The model under review builds one solid part; all positions refer to its coordinate system, in mm. Give positions to 0.01 mm unless a question says otherwise; leave off trailing zeros. Loops run counter-clockwise (first coordinate to the right, second up) from the corner with the lowest first, then second, coordinate; pieces in that order, holes last. Notation, with made-up numbers: (41, 57.25) -> (64, 57.25) arc R14 ccw to (64, 74.25) -> close; hole circle Ø3 at (-19.5, -33.75). An arc over 180 degrees is marked (long way). Write each question's results on one line, items separated by ' | '. Start each with the question number.
Q1. Insertion check: pin 1 Ø2.5 at (y, z) = (4, 0.5) entering from -X; pin 2 Ø4 at (x, y) = (116, 0) entering from -Z. Each pin has a flat end and moves straight along its axis. Give the tip position at first contact, or say it passes through.
Q2. Wall thickness on L1, parallel to X at y = 0, z = 3.35; L2, parallel to X at y = 1, z = 3.85; L3, parallel to Y at x = 116, z = 3.15: over which ranges is each line inside the solid? List them lowest first. Write a range as [from, to].
Q3. We need section A-A (z = 1.35). Write out the cut boundary in (x, y).
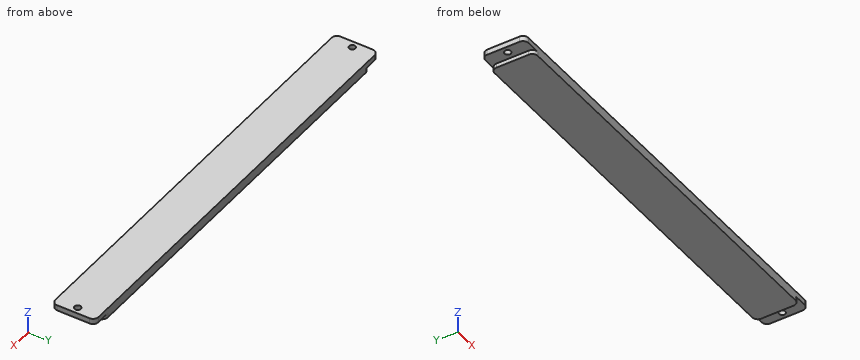
Autodesk Fusion 360 part; units mm, degrees
sketch "Sketch1" plane through (0, 0, 0) normal (0, 0, 1) x (1, 0, 0)
  circle A0 centre (-108.85, 8.85) radius 3
  circle A1 centre (-108.85, -8.85) radius 3
  circle A2 centre (108.85, 8.85) radius 3
  circle A3 centre (108.85, -8.85) radius 3
  line L0 (-128.9727, 0) -> (128.9727, 0) construction
  line L1 (0, 49.8209) -> (0, -49.8209) construction
  line L2 (-108.85, 11.85) -> (108.85, 11.85)
  line L3 (111.85, 8.85) -> (111.85, -8.85)
  line L4 (108.85, -11.85) -> (-108.85, -11.85)
  line L5 (-111.85, -8.85) -> (-111.85, 8.85)
  dimension "d1" = 6
  dimension "d2" = 6
  dimension "d3" = 6
  dimension "d4" = 6
  dimension "d5" = 17.7
  dimension "d6" = 217.7
  dimension "d50" = 23.7
  dimension "d51" = 223.7
extrude "Extrude1" add sketch "Sketch1" along normal blind 2.4
sketch "Sketch2" plane through (0, 0, 2.4) normal (0, 0, 1) x (-1, 0, 0)
  arc A0 (-108.85, 11.85) -> (-111.85, 8.85) centre (-108.85, 8.85) ccw
  line L0 (-111.85, 8.85) -> (-111.85, -8.85)
  arc A1 (-111.85, -8.85) -> (-108.85, -11.85) centre (-108.85, -8.85) ccw
  line L1 (-108.85, -11.85) -> (108.85, -11.85)
  arc A2 (108.85, -11.85) -> (111.85, -8.85) centre (108.85, -8.85) ccw
  line L2 (111.85, -8.85) -> (111.85, 8.85)
  arc A3 (111.85, 8.85) -> (108.85, 11.85) centre (108.85, 8.85) ccw
  line L3 (108.85, 11.85) -> (-108.85, 11.85)
  line L4 (150.244, 0) -> (144.5168, 0)
  line L5 (144.5168, 0) -> (-144.5168, 0) construction
  line L6 (0, -32.2256) -> (0, 32.2256) construction
  circle A4 centre (116.7, -8.85) radius 3
  circle A5 centre (116.7, 8.85) radius 3
  circle A6 centre (-116.7, -8.85) radius 3
  circle A7 centre (-116.7, 8.85) radius 3
  circle A8 centre (108.85, -8.85) radius 3
  circle A9 centre (108.85, 8.85) radius 3
  circle A10 centre (-108.85, -8.85) radius 3
  circle A11 centre (-108.85, 8.85) radius 3
  line L7 (119.7, -8.85) -> (119.7, 8.85)
  line L8 (116.7, 11.85) -> (-116.7, 11.85)
  line L9 (-119.7, 8.85) -> (-119.7, -8.85)
  line L10 (-116.7, -11.85) -> (-115.6655, -11.85)
  line L11 (-115.6655, -11.85) -> (116.7, -11.85)
  dimension "d9" = 6
  dimension "d10" = 6
  dimension "d11" = 6
  dimension "d12" = 6
  dimension "d13" = 6
  dimension "d14" = 6
  dimension "d15" = 6
  dimension "d16" = 6
  dimension "d18" = 7.85
extrude "Extrude2" add sketch "Sketch2" along normal blind 3
sketch "Sketch3" plane through (0, 0, 5.4) normal (0, 0, 1) x (-1, 0, 0)
  line L0 (-116.7, -11.85) -> (116.7, -11.85)
  arc A0 (116.7, -11.85) -> (119.7, -8.85) centre (116.7, -8.85) ccw
  line L1 (119.7, -8.85) -> (119.7, 8.85)
  arc A1 (119.7, 8.85) -> (116.7, 11.85) centre (116.7, 8.85) ccw
  line L2 (116.7, 11.85) -> (-116.7, 11.85)
  arc A2 (-116.7, 11.85) -> (-119.7, 8.85) centre (-116.7, 8.85) ccw
  line L3 (-119.7, 8.85) -> (-119.7, -8.85)
  arc A3 (-119.7, -8.85) -> (-116.7, -11.85) centre (-116.7, -8.85) ccw
  circle A4 centre (116, 0) radius 1.75
  circle A5 centre (-116, 0) radius 1.75
  line L4 (0, -34.4653) -> (0, -31.8477)
  line L5 (0, -31.8477) -> (0, 31.8477) construction
  dimension "d21" = 3.5
  dimension "d22" = 3.5
  dimension "d23" = 11.85
  dimension "d24" = 3.7
  dimension "d52" = 231.7
extrude "Extrude3" cut sketch "Sketch3" against normal blind 6 contours A4 | A5
equation "d2 = d1"
equation "d3 = d1"
equation "d4 = d1"
equation "d10 = d9"
equation "d11 = d9"
equation "d12 = d9"
equation "d14 = d13"
equation "d15 = d13"
equation "d16 = d13"
equation "d22 = d21"
Output:
1) pin 1: x = -111.85 | pin 2: z = 2.4
2) L1: [-119.7, -117.75], [-114.25, 114.25], [117.75, 119.7] | L2: [-119.7, -117.44], [-114.56, 114.56], [117.44, 119.7] | L3: [-11.85, -1.75], [1.75, 11.85]
3) outline: (-111.85, -8.85) arc R3 ccw to (-108.85, -11.85) -> (108.85, -11.85) arc R3 ccw to (111.85, -8.85) -> (111.85, 8.85) arc R3 ccw to (108.85, 11.85) -> (-108.85, 11.85) arc R3 ccw to (-111.85, 8.85) -> close
